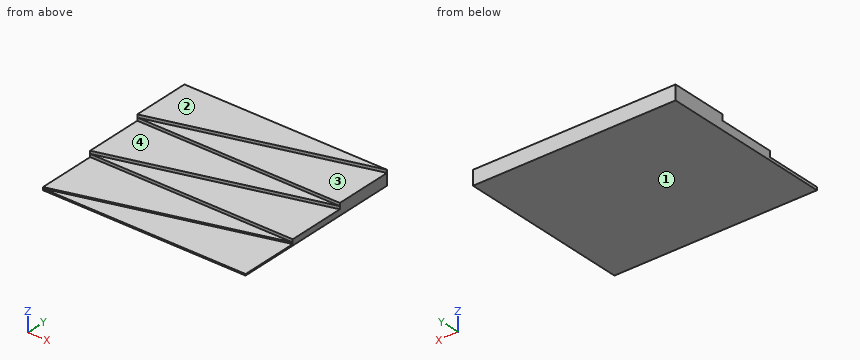
from build123d import *

# Parameters (mm, degrees)
F1_DEPTH = 0.5
F2_DEPTH = 1
F3_DEPTH = 2
F4_DEPTH = 3
F5_DEPTH = 4
F6_DEPTH = 5


with BuildPart() as f1:
    # F0 (on Top) → F1 (new body)
    with BuildSketch(Plane.XY):
        Polygon((36.676646, -130), (36.676646, -110), (-33.323354, -130), align=None)
    extrude(amount=F1_DEPTH)

    # F0 (on Top) → F2 (join)
    with BuildSketch(Plane.XY):
        Polygon((36.676646, -110), (-33.323354, -110), (-33.323354, -130), align=None)
    extrude(amount=F2_DEPTH)

    # F0 (on Top) → F3 (join)
    with BuildSketch(Plane.XY):
        Polygon((36.676646, -110), (36.676646, -90), (-33.323354, -110), align=None)
    extrude(amount=F3_DEPTH)

    # F0 (on Top) → F4 (join)
    with BuildSketch(Plane.XY):
        Polygon((36.676646, -90), (-33.323354, -90), (-33.323354, -110), align=None)
    extrude(amount=F4_DEPTH)

    # F0 (on Top) → F5 (join)
    with BuildSketch(Plane.XY):
        Polygon((36.676646, -90), (36.676646, -70), (-33.323354, -90), align=None)
    extrude(amount=F5_DEPTH)

    # F0 (on Top) → F6 (join)
    with BuildSketch(Plane.XY):
        Polygon((36.676646, -70), (-33.323354, -70), (-33.323354, -90), align=None)
    extrude(amount=F6_DEPTH)


solid = f1.part
Source: CAD feature listing. Evaluate the final solid. Frame: model axes, mm. Face numbers are marked on the shaded views. A direction names the side the tool comes from. Round coordinates to 2 decimals unless told otherwise and drop trailing zeros. Write each loop counter-clockwise with the first axis right and the second up, starting at its lowest first coordinate (ties: lowest second). Pieces come first, ordered by that corner, then holes. Notation, with made-up numbers: M 89.25,49.5 L 115.25,49.5 A19 cw 115.25,84.5 Z; hole C 30.25,83 d6. An arc over 180 degrees is marked long. One line per item, written item: value. Start each with the question number.
Item 1: Section query C-C (x = -21.5). Return the cut outline in (y, z).
Item 2: Pin query (flat end, axial travel): pin 1 (16 mm diameter, centred on x = 13, y = -115.5, fed in from +Z); pin 2 (22 mm diameter, centred on x = 17, y = -124.5, fed in from +Z); pin 3 (3 mm diameter, centred on x = 11.5, y = -98.5, fed in from +Z). Return the tip coordinate at first contact, or that it passes through.
Item 3: Section query A-A (x = 27). Return the cut outline in (y, z).
Item 4: Section query D-D (y = -85). Return the cut outline in (x, z), plus the area to 4 significant figures.
Item 5: Set-up query: the marked faces 3 and 4. Return all of +Z, -Z, +X, -X, +Y, -Y with unobstructed straight access to the full face (end or side cutting, diameter ignored); none if empty.
Item 6: Section query B-B (y = -124). Return the cut outline in (x, z), plus the area to 3 significant figures.
Item 7: Ray query, L1, parallel to Z at x = -22, y = -127.5; L2, parallel to Y at x = -9, z = 1.55; L3, parallel to Z at x = 19, y = -115. Return the intervals inside material, ascending. Write a range as from..to.
Item 8: Mould query, pull axis Z, two halves, no side actions, for the marked faces 1 and 2. Classes: pulls with the +Z half, pulls with the -Z half, needs draft (parallel to the pull), parting line crosses it, or undercut.
Result set:
1. outline: M -130,0 L -70,0 L -70,5 L -86.62,5 L -86.62,4 L -90,4 L -90,3 L -106.62,3 L -106.62,2 L -110,2 L -110,1 L -126.62,1 L -126.62,0.5 L -130,0.5 Z
2. pin 1: stops at z = 2
2. pin 2: stops at z = 1
2. pin 3: stops at z = 3
3. outline: M -130,0 L -70,0 L -70,5 L -72.76,5 L -72.76,4 L -90,4 L -90,3 L -92.76,3 L -92.76,2 L -110,2 L -110,1 L -112.76,1 L -112.76,0.5 L -130,0.5 Z
4. outline: M -33.32,0 L 36.68,0 L 36.68,4 L -15.82,4 L -15.82,5 L -33.32,5 Z
4. area: 297.5 mm²
5. face 3: +Z, +X, -Y
5. face 4: +Z, +X, -X, -Y
6. outline: M -33.32,0 L 36.68,0 L 36.68,0.5 L -12.32,0.5 L -12.32,1 L -33.32,1 Z
6. area: 45.5 mm²
7. L1: z = 0..0.5
7. L2: y = -110..-70
7. L3: z = 0..1
8. face 1: pulls with the -Z half
8. face 2: pulls with the +Z half
